Read the model definition and answer for the solid it produces. Units are mm, in the model's axes. A direction names the side the tool comes from. Coordinates: 2 decimals unless noted, no trailing zeros. Write each loop counter-clockwise with the first axis right and the second up, starting at its lowest first coordinate (ties: lowest second). Pieces come first, ordered by that corner, then holes. Notation, with made-up numbers: M 20.25,76 L 51.25,76 A24 cw 51.25,109 Z; hole C 89,3 d10. An arc over 180 degrees is marked long. Use a Markdown table: item, result. Add a question column.
from build123d import *

# Parameters (mm, degrees)
SKETCH1_W             = 3
SKETCH1_H             = 10
BOSS_EXTRUDE1_DEPTH   = 18
BOSS_EXTRUDE1_2_DEPTH = 18
SKETCH2_W             = 20
SKETCH2_H             = 5
SKETCH2_H_2           = 15
BOSS_EXTRUDE2_DEPTH   = 3
SKETCH3_W             = 11
SKETCH3_H             = 3
CUT_EXTRUDE1_DEPTH    = 2


with BuildPart() as part:
    # Sketch1 → Boss-Extrude1 (new body)
    with BuildSketch(Plane(origin=(0, 0, 0), x_dir=(1, 0, 0), z_dir=(0, 1, 0))):
        with Locations((-4, 0)):
            Rectangle(SKETCH1_W, SKETCH1_H)
    extrude(amount=BOSS_EXTRUDE1_DEPTH)



with BuildPart() as body_2:
    # Sketch1 → Boss-Extrude1 2 (new body)
    with BuildSketch(Plane(origin=(0, 0, 0), x_dir=(1, 0, 0), z_dir=(0, 1, 0))):
        with Locations((4, 0)):
            Rectangle(SKETCH1_W, SKETCH1_H)
    extrude(amount=BOSS_EXTRUDE1_2_DEPTH)


with BuildPart() as part_1:
    add(part.part)

    add(body_2.part)  # Boss-Extrude2 merges body 2
    # Sketch2 → Boss-Extrude2 (add)
    with BuildSketch(Plane.XZ):
        with Locations((0, 10)):
            Rectangle(SKETCH2_W, SKETCH2_H)
        Rectangle(SKETCH2_W, SKETCH2_H_2)
    extrude(amount=BOSS_EXTRUDE2_DEPTH)

    # Sketch3 → Cut-Extrude1 (cut)
    with BuildSketch(Plane.XY.offset(5)):
        with Locations((0, 11.5)):
            Rectangle(SKETCH3_W, SKETCH3_H)
    extrude(amount=-CUT_EXTRUDE1_DEPTH, mode=Mode.SUBTRACT)


solid = part_1.part
Item 1: Determine the mould class of faces 1 (the flat face through (4, 9, -5)), 2 (the flat face through (0, -3, 3)), 3 (the flat face through (4, 13, 4)) for opening direction Y: pulls with the +Y half, pulls with the -Y half, needs draft (parallel to the pull), parting line crosses it, or undercut.
Item 2: Find section B-B on y = 5.5. Give the vertices of the cut face in (x, z), then the cut area to 3 significant figures.
Item 3: Consider probe 1 along X at (y, z) = (8.5, 1); probe 2 along Y at (x, z) = (0.5, 8); probe 3 along Z at (x, y) = (4, 8.75). Determine where each line is inside the solid, lowest interval first.
Item 4: Find section D-D on x = 0.25. Give the vertices of the cut face in (y, z).
Item 5: Each of these flat-tipped pins is pushed along its axis until it touches: pin 1 (1.5 mm diameter, centred on x = 4, y = 5, fed in from -Z); pin 2 (1.5 mm diameter, centred on x = -5, z = 10.5, fed in from +Y); pin 3 (6 mm diameter, centred on y = 11.5, z = -4.5, fed in from -X). Where does it stop, or does it pass through?
Item 6: For faces 4 (the flat face through (5.5, 9, 0)), 5 (the flat face through (4, 15, 5)), 6 (the flat face through (-2.5, 9, 0)), determine the directions among +Z, -Z, +X, -X, +Y, -Y from which every point of the face is accessible in a straight line to the end or side of a thin tool.
Item 7: Find section A-A on z = 3.5. Give the vertices of the cut face in (x, y).
Item 8: Find section C-C on z = 1.25. Give the vertices of the cut face in (x, y).
Geometry says:
| question | item | result |
|---|---|---|
| 1 | face 1 | needs draft |
| 1 | face 2 | pulls with the -Y half |
| 1 | face 3 | undercut |
| 2 | outline | M -5.5,-5 L -2.5,-5 L -2.5,5 L -5.5,5 Z; M 2.5,-5 L 5.5,-5 L 5.5,5 L 2.5,5 Z |
| 2 | area | 60.0 mm2 |
| 3 | probe 1 | x = -5.5 to -2.5, 2.5 to 5.5 |
| 3 | probe 2 | y = -3 to 0 |
| 3 | probe 3 | z = -5 to 5 |
| 4 | outline | M -3,-7.5 L 0,-7.5 L 0,12.5 L -3,12.5 Z |
| 5 | pin 1 | stops at z = -5 |
| 5 | pin 2 | stops at y = 0 |
| 5 | pin 3 | stops at x = -5.5 |
| 6 | face 4 | +Z, -Z, +X, +Y |
| 6 | face 5 | +Z, +X, -X, +Y |
| 6 | face 6 | +Z, -Z, +Y |
| 7 | outline | M -10,-3 L 10,-3 L 10,0 L 5.5,0 L 5.5,10 L 2.5,10 L 2.5,0 L -2.5,0 L -2.5,10 L -5.5,10 L -5.5,0 L -10,0 Z; M -5.5,13 L -2.5,13 L -2.5,18 L -5.5,18 Z; M 2.5,13 L 5.5,13 L 5.5,18 L 2.5,18 Z |
| 8 | outline | M -10,-3 L 10,-3 L 10,0 L 5.5,0 L 5.5,18 L 2.5,18 L 2.5,0 L -2.5,0 L -2.5,18 L -5.5,18 L -5.5,0 L -10,0 Z |
